Work out the finished part from the listing and answer in its coordinate system (mm). A direction names the side the tool comes from. Give positions to 0.01 mm unless a question says otherwise; leave off trailing zeros. Loops run counter-clockwise (first coordinate to the right, second up) from the corner with the lowest first, then second, coordinate; pieces in that order, holes last. Notation, with made-up numbers: M 19,-17 L 40,-17 A20 ccw 40,-11 Z; hole C 46.25,30 d2. An arc over 180 degrees is marked long. Answer in a Markdown table with one row per item. Add a question column.
from build123d import *

# Parameters (mm, degrees)
F0_W     = 42
F0_H     = 32.8
F0_R     = 5
F1_DEPTH = 14
F2_W     = 12
F2_H     = 26.8
F3_DEPTH = 14
F4_R     = 2.5
F5_DEPTH = 25.4


with BuildPart() as f1:
    # F0 (on Top) → F1 (new body)
    with BuildSketch(Plane.XY):
        with Locations((21, 16.4)):
            Rectangle(F0_W, F0_H)
        with Locations((21, 20)):
            Circle(F0_R, mode=Mode.SUBTRACT)
    extrude(amount=F1_DEPTH)

    # F2 (on face) → F3 (cut)
    with BuildSketch(Plane.XY.offset(14)):
        with Locations((6, 19.4)):
            Rectangle(F2_W, F2_H)
        with Locations((36, 19.4)):
            Rectangle(F2_W, F2_H)
    extrude(amount=-F3_DEPTH, mode=Mode.SUBTRACT)

    # F4 (on face) → F5 (cut)
    with BuildSketch(Plane.XZ):
        with Locations((5, 7)):
            Circle(F4_R)
        with Locations((37, 7)):
            Circle(F4_R)
    extrude(amount=-F5_DEPTH, mode=Mode.SUBTRACT)


solid = f1.part
(1) Which of the six approach directions +Z, -Z, +X, -X, +Y, -Y give full straight-line access (tool end or side, diameter ignored) to faces 1 (the face through (21, 32.8, 7)), 2 (the face through (30, 19, 7)), 3 (the face through (7, 6, 9))?
(2) Each of these flat-tipped pins is pushed along its axis until it touches: P1, Ø3, axis at x = 37, z = 7, coming from the +Y side; P2, Ø1, axis at x = 37.5, z = 4.5, coming from the +Y side; P3, Ø4, axis at y = 17.5, z = 9.5, coming from the -X side. Where does it stop, or does it pass through?
(3) Section D-D, the plane z = 12.5 is taken. Determine the outline of the cut face in (x, y).
(4) The mould has two halves that part along X. Classify faces 4 (the face through (39.31, 2.96, 6.04)), 5 (the face through (34.6, 6, 5.5)), 6 (the face through (19.92, 15.12, 6.9)), 7 (the face through (12, 19, 7)): pulls with the +X half, pulls with the -X half, needs draft (parallel to the pull), parting line crosses it, or undercut.
(5) Section C-C, the plane x = 37 is taken. Determine the outline of the cut face in (y, z), and give its area (3 significant figures).
(6) Consider line 1 along Z through (x, y) = (5, 3.7); line 2 along Y through (x, z) = (21, 7); line 3 along X through (y, z) = (29, 6.75). Determine where each line is inside the solid, lowest interval first. Write a range as from..to.
(7) Section B-B, the plane y = 20 is taken. Determine the outline of the cut face in (x, z), and give its area (3 significant figures).
(8) Section A-A, the plane z = 7 is taken. Determine the outline of the cut face in (x, y).
Numbers:
| question | item | result |
|---|---|---|
| 1 | face 1 | +Z, -Z, +X, -X, +Y |
| 1 | face 2 | +Z, -Z, +X, +Y |
| 1 | face 3 | +Z, -Z, -X, +Y |
| 2 | P1 | passes through |
| 2 | P2 | stops at y = 6 |
| 2 | P3 | stops at x = 12 |
| 3 | outline | M 0,0 L 42,0 L 42,6 L 30,6 L 30,32.8 L 12,32.8 L 12,6 L 0,6 Z; hole C 21,20 d10 |
| 4 | face 4 | undercut |
| 4 | face 5 | needs draft |
| 4 | face 6 | undercut |
| 4 | face 7 | pulls with the -X half |
| 5 | outline | M 0,0 L 6,0 L 6,4.5 L 0,4.5 Z; M 0,9.5 L 6,9.5 L 6,14 L 0,14 Z |
| 5 | area | 54.0 mm² |
| 6 | line 1 | z = 0..4.5, 9.5..14 |
| 6 | line 2 | y = 0..15, 25..32.8 |
| 6 | line 3 | x = 12..30 |
| 7 | outline | M 12,0 L 16,0 L 16,14 L 12,14 Z; M 26,0 L 30,0 L 30,14 L 26,14 Z |
| 7 | area | 112 mm² |
| 8 | outline | M 0,0 L 2.5,0 L 2.5,6 L 0,6 Z; M 7.5,0 L 34.5,0 L 34.5,6 L 30,6 L 30,32.8 L 12,32.8 L 12,6 L 7.5,6 Z; M 39.5,0 L 42,0 L 42,6 L 39.5,6 Z; hole C 21,20 d10 |
